Print and shaded views of the part. All mm, measured from the part's lowest x, y and z. Coordinates: 2 decimals unless noted, no trailing zeros. Order: outer loops, then holes, each group sorted by start corner. A loop starts at its lowest first (then second) coordinate and runs counter-clockwise, first axis right, second up. Notation, with made-up numbers: (-7, -39.5) - (27, -39.5) arc R33 ccw to (27, -0.5) - close; hole circle Ø8 at (-6.75, 65.5). An arc over 180 degrees is marked (long way). Write each question's results on one line, items separated by ' | '.
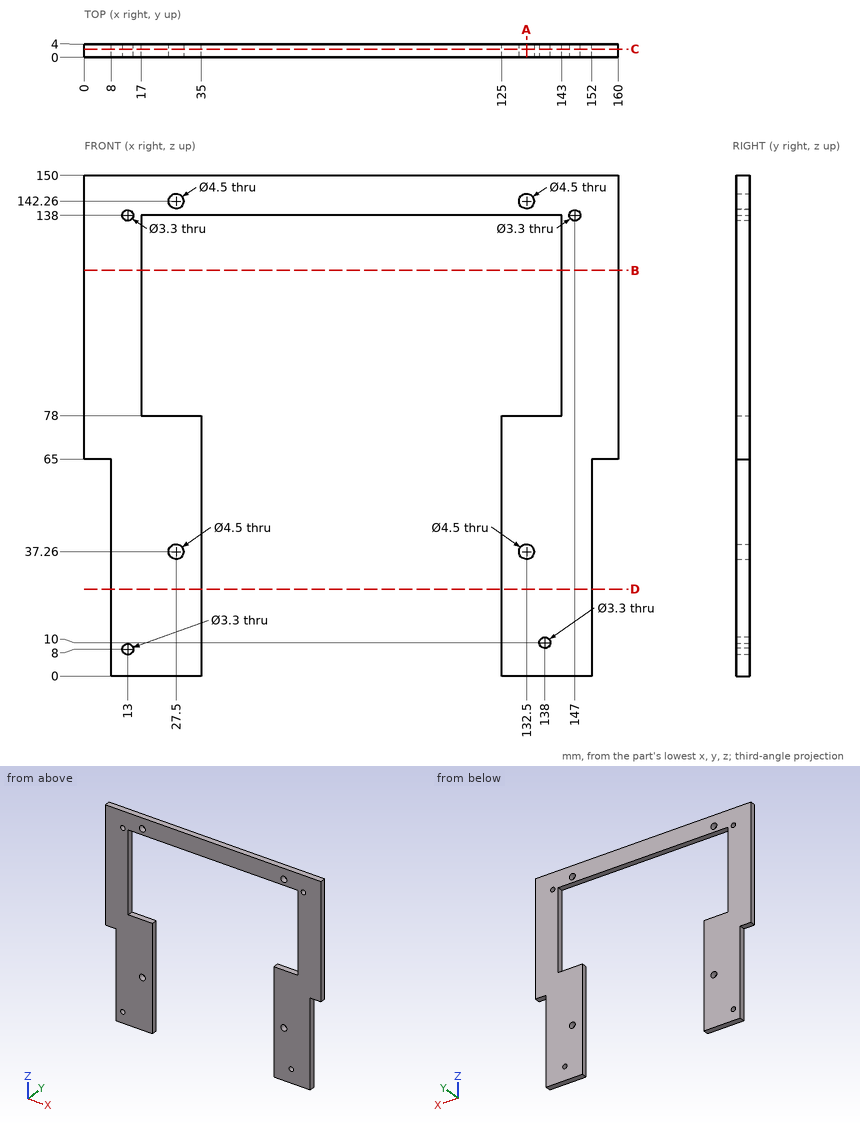
1. Band-saw the part on B-B on z = 121.5. Give the cut face in (x, y), then the cut area to 3 significant figures.
Solved:
outline: (0, 0) - (17, 0) - (17, 4) - (0, 4) - close; (143, 0) - (160, 0) - (160, 4) - (143, 4) - close | area: 136 mm2
2. Band-saw the part on D-D on z = 26. Give the cut face in (x, y), then the cut area to 3 significant figures.
Solved:
outline: (8, 0) - (35, 0) - (35, 4) - (8, 4) - close; (125, 0) - (152, 0) - (152, 4) - (125, 4) - close | area: 216 mm2
3. Drop flat-ended pins along their axis: pin 1 Ø2.5 at (x, z) = (13, 8) entering from +Y; pin 2 Ø1.2 at (x, y) = (156, 1.5) entering from -Z; pin 3 Ø1 at (x, y) = (55.5, 3.5) entering from -Z; pin 4 Ø2 at (y, z) = (2.5, 44) entering from -X. Give the stop position or say it passes through.
Solved:
pin 1: passes through | pin 2: stops at z = 65 | pin 3: stops at z = 138 | pin 4: stops at x = 8
4. Probe line 1 (Z direction, x = 138, y = 1.35); line 2 (Z direction, x = 13, y = 1.3); line 3 (Z direction, x = 132.5, y = 2.9). List the from-to ranges inside material, lowest first.
Solved:
line 1: z = 0 to 8.35, 11.65 to 78, 138 to 150 | line 2: z = 0 to 6.35, 9.65 to 136.35, 139.65 to 150 | line 3: z = 0 to 35.01, 39.51 to 78, 138 to 140.01, 144.51 to 150
5. Band-saw the part on C-C on y = 2.45. Give the number of separate pieces and of enclosed holes in the cut face, then the cut area to 3 significant figures.
Solved:
separate pieces: 1 | enclosed holes: 8 | area: 8,280 mm2
6. Band-saw the part on A-A on x = 132.5. Give the cut face in (y, z), then the cut area to 3 significant figures.
Solved:
outline: (0, 0) - (4, 0) - (4, 35.01) - (0, 35.01) - close; (0, 39.51) - (4, 39.51) - (4, 78) - (0, 78) - close; (0, 138) - (4, 138) - (4, 140.01) - (0, 140.01) - close; (0, 144.51) - (4, 144.51) - (4, 150) - (0, 150) - close | area: 324 mm2
